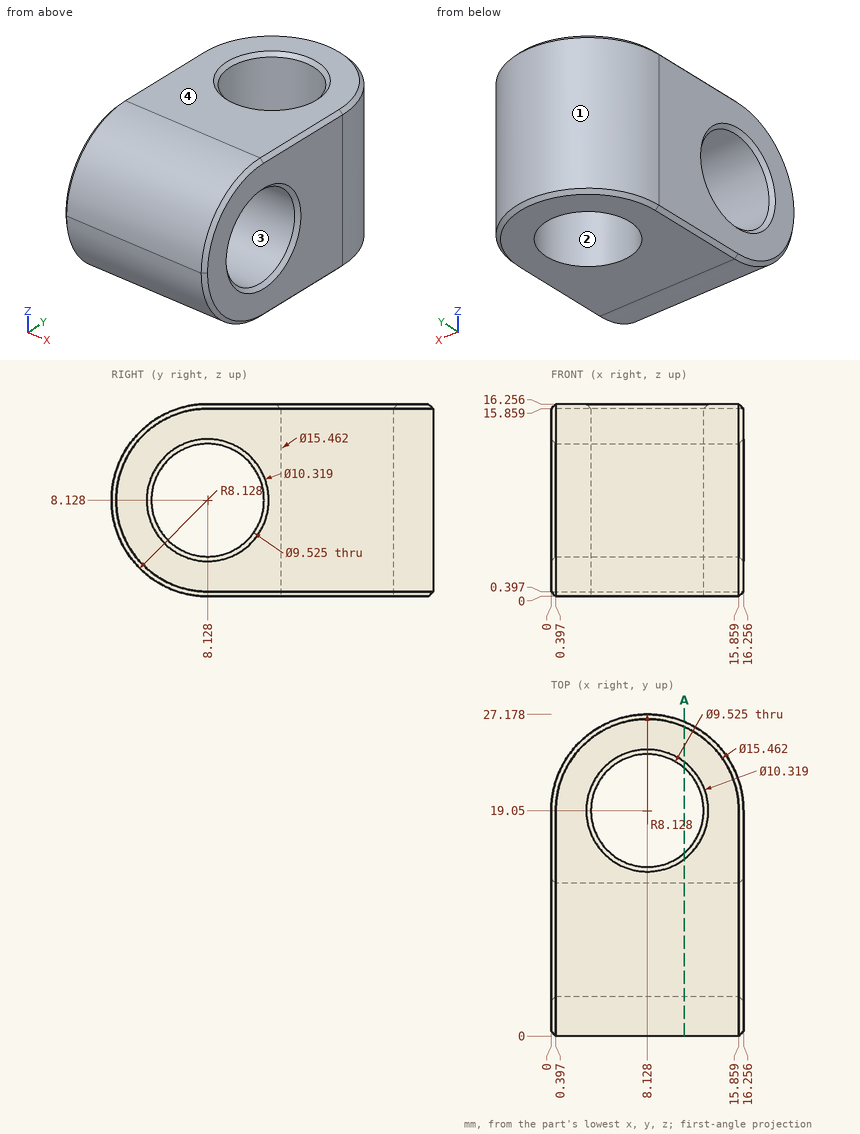
Study the drawing (mm; zero at the part's minimum x, y, z) and answer. Give positions to 0.01 mm unless a question says otherwise; leave off trailing zeros. Write item = value, one per line. Start each with the question number.
(1) Find section A-A on x = 11.25. Give the number of separate pieces and of enclosed holes in the cut face, and give its area (3 significant figures).
(2) Find the intervals of material crossed by probe 1 along Y at (x, z) = (11, 8.25); probe 2 along Y at (x, z) = (6.5, 12) (1 decimal); probe 3 along X at (y, z) = (17, 12.5), in increasing order. Write a range as from..to.
(3) Given pin 1 Ø1.5 at (x, z) = (6.5, 13) entering from -Y; pin 2 Ø5.5 at (x, y) = (8.128, 19.05) entering from +Z; pin 3 Ø1.5 at (y, z) = (23, 14.5) entering from +X, each flat-ended and moving along its own axis, determine where each tip first touches the part or whether it passes through.
(4) The mould has two halves that part along Y. Classify the marked faces 1, 2, 3 and 4: +Y half, -Y half, draft (parallel to the pull), parting line (faces both ways), or undercut.
From the geometry:
q1.separate_pieces = 2
q1.enclosed_holes = 1
q1.area = 215 mm^2
q2.probe_1 = 0..3.37, 12.89..15.25, 22.85..26.65
q2.probe_2 = 1..5.4, 10.9..14.6, 23.5..27
q2.probe_3 = 0..3.83, 12.43..16.26
q3.pin_1 = 1.12
q3.pin_2 = through
q3.pin_3 = 15.6
q4.face_1 = +Y half
q4.face_2 = undercut
q4.face_3 = undercut
q4.face_4 = draft
